Check sheet for the drawn part. Datum: minimum x, y, z corner. Units: mm. A direction names the side the tool comes from. Coordinates: 2 decimals unless noted, no trailing zeros. Loops run counter-clockwise (first coordinate to the right, second up) from the corner with the lowest first, then second, coordinate; pieces in that order, holes last. Notation, with made-up numbers: (31, 58) -> (49, 58) arc R24 cw to (49, 97) -> close; hole circle Ø4 at (34.25, 13.5). An arc over 180 degrees is marked (long way). Use CSV: the item, a comma, the result in double quotes. Start each with the question number.
1. Sectioned sample at C-C, the plane z = 6.43. Record the cut outline in (x, y) (3 decimals).
2. Sectioned sample at A-A, the plane x = 90. Record the cut outline in (y, z) (3 decimals), and give its area (3 significant figures).
3. Gauge pin test, flat end, axial feed: pin 1 (1.5 mm diameter, centred on x = 25.5, z = 13, fed in from -Y). Record the tip position at first contact, or that the pin passes through.
4. Sectioned sample at B-B, the plane y = 4.25. Record the cut outline in (x, z) (3 decimals), and give its area (3 significant figures).
5. Set-up check for the marked faces 4, 5 and 6: record each of +Z, -Z, +X, -X, +Y, -Y from which the full face is reachable in a straight line by a thin tool's end or side.
6. Release check for a two-part mould opening along Z. For the marked faces 1, 2 and 3 record: pulls with the +Z half, pulls with the -Z half, needs draft (parallel to the pull), parting line crosses it, or undercut.
7. Thickness scan on L1, parallel to Z at x = 90, y = 20.25 (3 decimals); L2, parallel to Z at x = 82, y = 11.25 (3 decimals); L3, parallel to X at y = 7.25, z = 55.5 (3 decimals). Record the ranges inside material, lowest first.
8. Sectioned sample at D-D, the plane y = 23.25. Count the separate pieces of the cut face and the enclosed holes in it, and give its area (3 significant figures).
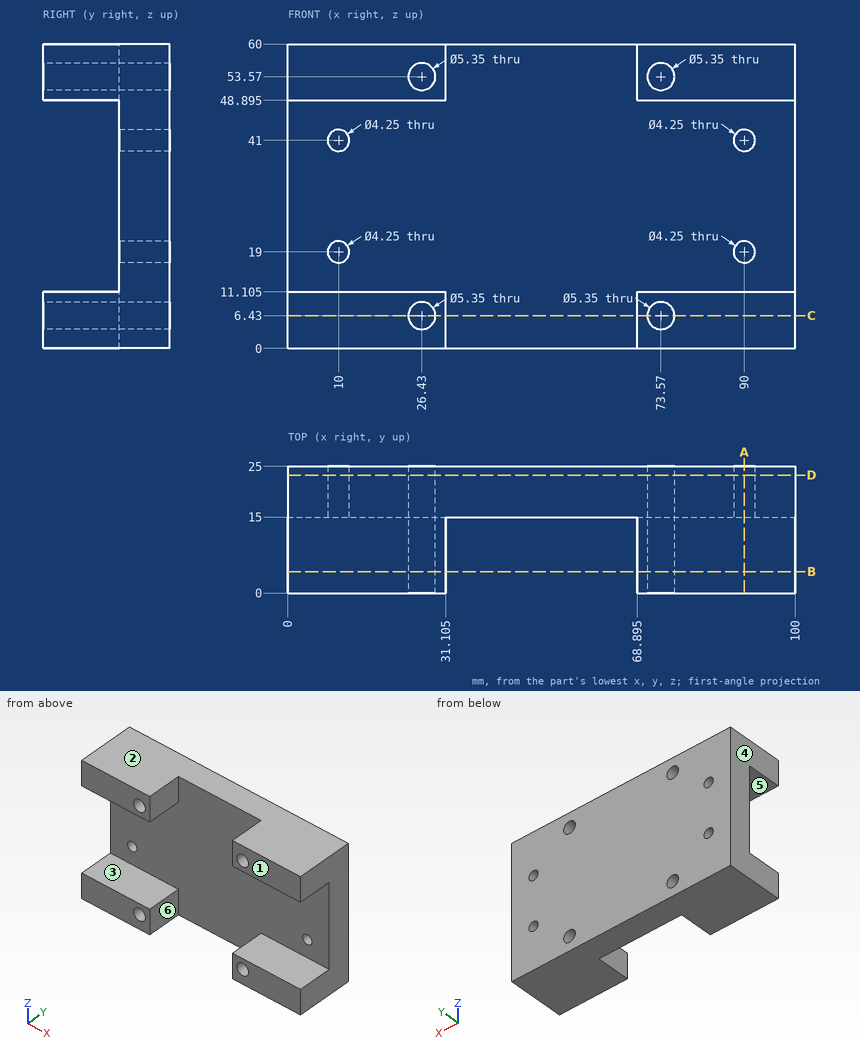
Completed:
1,outline,"(0, 0) -> (23.755, 0) -> (23.755, 25) -> (0, 25) -> close; (29.105, 0) -> (31.105, 0) -> (31.105, 15) -> (68.895, 15) -> (68.895, 0) -> (70.895, 0) -> (70.895, 25) -> (29.105, 25) -> close; (76.245, 0) -> (100, 0) -> (100, 25) -> (76.245, 25) -> close"
2,outline,"(0, 0) -> (25, 0) -> (25, 16.875) -> (15, 16.875) -> (15, 11.105) -> (0, 11.105) -> close; (0, 48.895) -> (15, 48.895) -> (15, 43.125) -> (25, 43.125) -> (25, 60) -> (0, 60) -> close; (15, 21.125) -> (25, 21.125) -> (25, 38.875) -> (15, 38.875) -> close"
2,area,"848 mm²"
3,pin 1,"y = 15"
4,outline,"(0, 0) -> (31.105, 0) -> (31.105, 11.105) -> (0, 11.105) -> close; (0, 48.895) -> (31.105, 48.895) -> (31.105, 60) -> (0, 60) -> close; (68.895, 0) -> (100, 0) -> (100, 11.105) -> (68.895, 11.105) -> close; (68.895, 48.895) -> (100, 48.895) -> (100, 60) -> (68.895, 60) -> close; hole circle Ø5.35 at (26.43, 6.43); hole circle Ø5.35 at (26.43, 53.57); hole circle Ø5.35 at (73.57, 6.43); hole circle Ø5.35 at (73.57, 53.57)"
4,area,"1,290 mm²"
5,face 4,"+Z, -Z, -X, +Y, -Y"
5,face 5,"+X, -X, -Y"
5,face 6,"+Z, -Z, -Y"
6,face 1,"needs draft"
6,face 2,"pulls with the +Z half"
6,face 3,"undercut"
7,L1,"0 to 16.875, 21.125 to 38.875, 43.125 to 60"
7,L2,"0 to 11.105, 48.895 to 60"
7,L3,"0 to 24.578, 28.282 to 31.105, 68.895 to 71.718, 75.422 to 100"
8,separate pieces,"1"
8,enclosed holes,"8"
8,area,"5,850 mm²"
